```python
from build123d import *

# Parameters (mm, degrees)
F0_W     = 60
F0_H     = 60
F1_DEPTH = 2
F2_W     = 5
F2_H     = 25
F3_DEPTH = 40
F4_DEPTH = 40
F5_R     = 12.49999
F7_D     = 5
F9_D     = 4
F9_DEPTH = 15
F9_TIP   = 1.2017212381


# Not quite as in the source:
# - a fillet or chamfer is up to 0.001 mm smaller than in the source, because OpenCascade refuses the exact size


with BuildPart() as f1:
    # F0 (on Top) → F1 (new body)
    with BuildSketch(Plane.XY):
        with Locations((35.6504749941, -30)):
            Rectangle(F0_W, F0_H)
    extrude(amount=F1_DEPTH)

    # F2 (on face) → F3 (join)
    with BuildSketch(Plane.XY.offset(2)):
        with Locations((19.6504749941, -30)):
            Rectangle(F2_W, F2_H)
    extrude(amount=F3_DEPTH)

    # F2 (on face) → F4 (join)
    with BuildSketch(Plane.XY.offset(2)):
        with Locations((51.6504749941, -30)):
            Rectangle(F2_W, F2_H)
    extrude(amount=F4_DEPTH)

    # F5 (radius 12.5 in the source; OpenCascade refuses exactly that, so slightly less here)
    f5_edges = [f1.edges().sort_by_distance(p)[0] for p in [
        (19.650475, -42.5, 42),
        (51.650475, -42.5, 42),
        (51.650475, -17.5, 42),
        (19.650475, -17.5, 42),
    ]]
    fillet(f5_edges, radius=F5_R)

    # F7 (through all)
    with Locations(Plane(origin=(17.1504749941, 0, 0), x_dir=(0, -1, 0), z_dir=(-1, 0, 0))):
        with Locations((30, 26.8072411418)):
            Hole(F7_D / 2)

    # F9
    with Locations(Plane.XY.offset(2)):
        with Locations((13.6504749941, -8), (13.6504749941, -52), (57.6504749941, -52), (57.6504749941, -8)):
            Hole(F9_D / 2, depth=F9_DEPTH)
            with Locations((0, 0, -(F9_DEPTH + F9_TIP / 2))):  # 118° drill point
                Cone(0, F9_D / 2, F9_TIP, mode=Mode.SUBTRACT)


solid = f1.part
```
Check sheet for the modelled part. Datum: model origin and axes. Units: mm. A direction names the side the tool comes from. Round coordinates to 2 decimals unless told otherwise and drop trailing zeros. Order: outer loops, then holes, each group sorted by start corner. A loop starts at its lowest first (then second) coordinate and runs counter-clockwise, first axis right, second up. Notation, with made-up numbers: (37, 32.5) - (86, 32.5) arc R22 ccw to (86, 57.5) - close; hole circle Ø6 at (70, -3.5). An arc over 180 degrees is marked (long way). Write item = value, one per line.
Q1. Section check B-B (z = 18). Record the boundary of the cut face in (x, y), and give its area (3 significant figures).
Computed:
outline = (17.15, -42.5) - (22.15, -42.5) - (22.15, -17.5) - (17.15, -17.5) - close; (49.15, -42.5) - (54.15, -42.5) - (54.15, -17.5) - (49.15, -17.5) - close
area = 250 mm^2
Q2. Go/stop test with flat-tipped pins: pin 1 (2 mm diameter, centred on x = 41.5, y = -34, fed in from -Z); pin 2 (2.5 mm diameter, centred on x = 19.5, z = 9, fed in from -Y); pin 3 (2.5 mm diameter, centred on x = 20, z = 13, fed in from +Y); pin 4 (12.5 mm diameter, centred on y = -26, z = 29, fed in from +X). Record where each tip stops, or that it passes through.
Computed:
pin_1 = 0
pin_2 = -42.5
pin_3 = -17.5
pin_4 = 54.15
Q3. Section check D-D (z = 34.5). Record the boundary of the cut face in (x, y).
Computed:
outline = (17.15, -41.46) - (22.15, -41.46) - (22.15, -18.54) - (17.15, -18.54) - close; (49.15, -41.46) - (54.15, -41.46) - (54.15, -18.54) - (49.15, -18.54) - close
Q4. Thickness scan on line 1 along X through (y, z) = (-20.5, 23.5); line 2 along Z through (x, y) = (53, -30); line 3 along Y through (x, z) = (53, 13). Record the ranges inside material, lowest first.
Computed:
line_1 = 17.15 to 22.15, 49.15 to 54.15
line_2 = 0 to 24.31, 29.31 to 42
line_3 = -42.5 to -17.5
Q5. Section check A-A (y = -52). Record the boundary of the cut face in (x, z), and give its area (3 significant figures).
Computed:
outline = (5.65, 0) - (11.65, 0) - (11.65, 2) - (5.65, 2) - close; (15.65, 0) - (55.65, 0) - (55.65, 2) - (15.65, 2) - close; (59.65, 0) - (65.65, 0) - (65.65, 2) - (59.65, 2) - close
area = 104 mm^2
Q6. Tool access check on faces 4 (the face through (52, -42.5, 16)), 5 (the face through (17.15, -30, 22)), 6 (the face through (20, -17.5, 16)). Record the directions out of +Z, -Z, +X, -X, +Y, -Y that give a thin tool (end or side, any length) a straight path to the whole face; none if there is none.
Computed:
face_4 = +Z, +X, -X, -Y
face_5 = +Z, -X, +Y, -Y
face_6 = +Z, +X, -X, +Y
Q7. Section check C-C (x = 58.5). Record the boundary of the cut face in (y, z).
Computed:
outline = (-60, 0) - (-53.81, 0) - (-53.81, 2) - (-60, 2) - close; (-50.19, 0) - (-9.81, 0) - (-9.81, 2) - (-50.19, 2) - close; (-6.19, 0) - (0, 0) - (0, 2) - (-6.19, 2) - close
Q8. Draft check along X on faces 1 (the face through (11.743, -7.399, 0.986)), 2 (the face through (54.15, -30, 22)), 3 (the face through (51.685, -21.065, 38.241)). Enter one of: pulls with the +X half, pulls with the -X half, needs draft (parallel to the pull), parting line crosses it, or undercut.
Computed:
face_1 = undercut
face_2 = pulls with the +X half
face_3 = needs draft
